For this review, use the dimensioned drawing (mm, ordinates from the lowest corner) and the shaded views. Round coordinates to 2 decimals unless told otherwise and drop trailing zeros. Write each loop counter-clockwise with the first axis right and the second up, starting at its lowest first coordinate (ties: lowest second). Pieces come first, ordered by that corner, then holes.
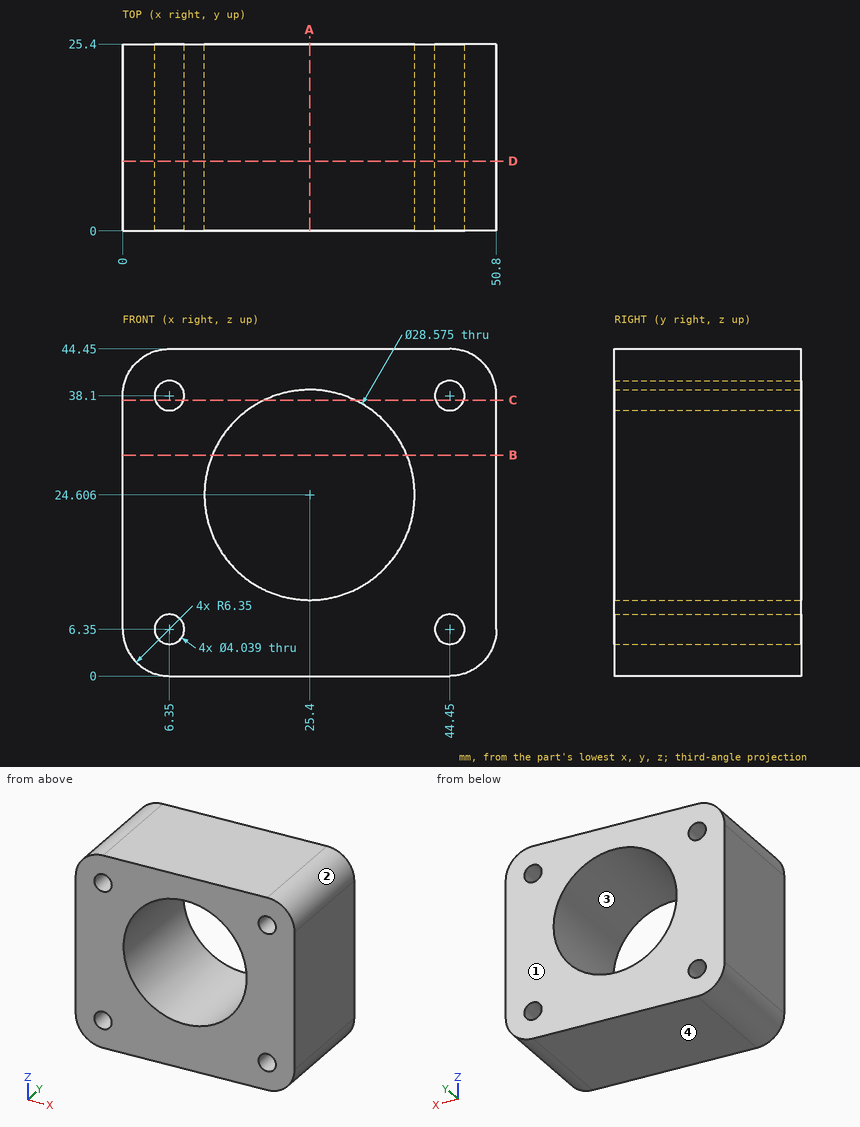
1) For P1, Ø2.5, axis at x = 44.45, z = 6.35, coming from the -Y side (3 decimals), flat-tipped, find the tip position at first contact; note if it passes through.
2) Add section A-A on x = 25.4. State the section outline as (y, z) points, and give its area (3 significant figures).
3) The part is to be moulded in two halves that separate along Z. For the marked faces 1, 2, 3 and 4, say which applies: pulls with the +Z half, pulls with the -Z half, needs draft (parallel to the pull), parting line crosses it, or undercut.
4) For line 1 along Z through (x, y) = (44.45, 20.25); line 2 along X through (y, z) = (7.5, 24.5); line 3 along Z through (x, y) = (6, 2.25), list the stretches that pass through material, from the lowest coordinate up.
5) Add section C-C on z = 37.5. State the section outline as (x, y) points (1 decimal).
6) Add section B-B on z = 30. State the section outline as (x, y) points.
7) Add section D-D on y = 9.5. Count the separate pieces of the cut face and the enclosed holes in it, and give its area (3 significant figures).
Computed:
1. P1: passes through
2. outline: (0, 0) - (25.4, 0) - (25.4, 10.32) - (0, 10.32) - close; (0, 38.89) - (25.4, 38.89) - (25.4, 44.45) - (0, 44.45) - close
2. area: 403 mm2
3. face 1: needs draft
3. face 2: pulls with the +Z half
3. face 3: undercut
3. face 4: pulls with the -Z half
4. line 1: z = 0 to 4.33, 8.37 to 36.08, 40.12 to 44.45
4. line 2: x = 0 to 11.11, 39.69 to 50.8
4. line 3: z = 0.01 to 4.36, 8.34 to 36.11, 40.09 to 44.44
5. outline: (0, 0) - (4.4, 0) - (4.4, 25.4) - (0, 25.4) - close; (8.3, 0) - (19.2, 0) - (19.2, 25.4) - (8.3, 25.4) - close; (31.6, 0) - (42.5, 0) - (42.5, 25.4) - (31.6, 25.4) - close; (46.4, 0) - (50.8, 0) - (50.8, 25.4) - (46.4, 25.4) - close
6. outline: (0, 0) - (12.17, 0) - (12.17, 25.4) - (0, 25.4) - close; (38.63, 0) - (50.8, 0) - (50.8, 25.4) - (38.63, 25.4) - close
7. separate pieces: 1
7. enclosed holes: 5
7. area: 1,530 mm2
